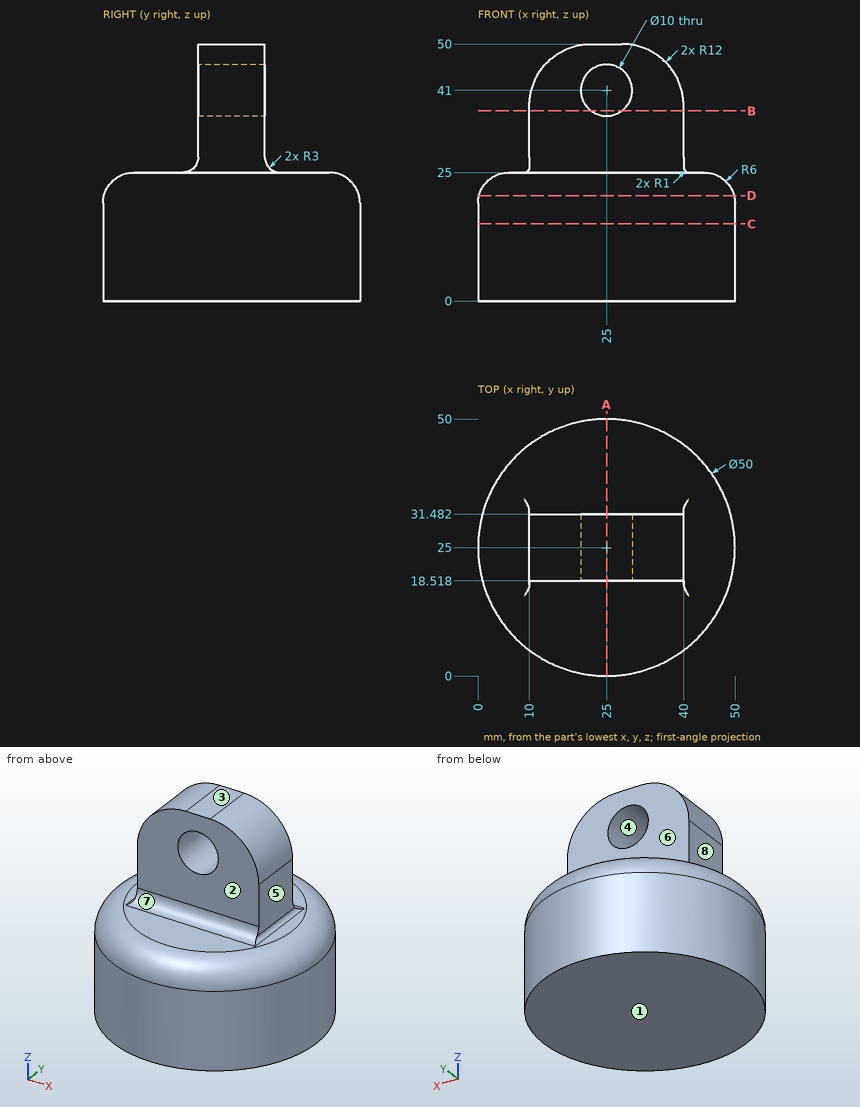
Check sheet for the drawn part. Datum: minimum x, y, z corner. Units: mm. A direction names the side the tool comes from. Give positions to 0.01 mm unless a question says otherwise; leave off trailing zeros. Loops run counter-clockwise (first coordinate to the right, second up) from the corner with the lowest first, then second, coordinate; pieces in that order, holes last. Notation, with made-up numbers: M 39.5,-25 L 52.5,-25 A11 ccw 52.5,-10 Z; hole C 24,-35.5 d10. An arc over 180 degrees is marked long. Return JSON: item names as keys, results as strings.
1) Tool access check on the marked faces 5, 6, 7 and 8. Record the directions out of +Z, -Z, +X, -X, +Y, -Y that give a thin tool (end or side, any length) a straight path to the whole face; none if there is none.
Findings:
{"face 5": "+Z, +X, +Y, -Y", "face 6": "+Z, +X, -X, +Y", "face 7": "+Z, +X, -X, -Y", "face 8": "+Z, -X, +Y, -Y"}
2) Mould release check, pull along Z, two halves, no side actions. Record for the marked faces 1, 2, 3 and 4: released by +Z, released by -Z, zero draft, split by the parting line, or undercut.
Findings:
{"face 1": "released by -Z", "face 2": "zero draft", "face 3": "released by +Z", "face 4": "undercut"}
3) Section check C-C, the plane z = 15. Enter the section's corners in (x, y), and give its area (3 significant figures).
Findings:
{"outline": "C 25,25 d50", "area": "1,960 mm2"}
4) Gauge pin test, flat ends, axial feed: P1, Ø12, axis at y = 15.5, z = 40.5, coming from the +X side; P2, Ø11, axis at x = 31.5, z = 38, coming from the +Y side; P3, Ø10, axis at x = 36, y = 27.5, coming from the -Z side; P4, Ø8, axis at x = 25, z = 41, coming from the -Y side. Record the tip position at first contact, or that the pin passes through.
Findings:
{"P1": "stops at x = 40", "P2": "stops at y = 31.48", "P3": "stops at z = 0", "P4": "passes through"}
5) Section check A-A, the plane x = 25. Enter the section's corners in (y, z).
Findings:
{"outline": "M 0,0 L 50,0 L 50,19 A6 ccw 44,25 L 34.48,25 A3 cw 31.48,28 L 31.48,36 L 18.52,36 L 18.52,28 A3 cw 15.52,25 L 6,25 A6 ccw 0,19 Z; M 18.52,46 L 31.48,46 L 31.48,50 L 18.52,50 Z"}
6) Section check D-D, the plane z = 20.5. Enter the section's corners in (x, y).
Findings:
{"outline": "C 25,25 d49.62"}
7) Material ranges on L1, parallel to X at y = 24.75, z = 41; L2, parallel to Y at x = 25, z = 2.5; L3, parallel to Y at x = 33.5, z = 33, recorded low to high. Write a range as [from, to].
Findings:
{"L1": "x = [10.38, 20], [30, 39.62]", "L2": "y = [0, 50]", "L3": "y = [18.52, 31.48]"}
8) Section check B-B, the plane z = 37. Enter the section's corners in (x, y).
Findings:
{"outline": "M 10,18.52 L 22,18.52 L 22,31.48 L 10,31.48 Z; M 28,18.52 L 40,18.52 L 40,31.48 L 28,31.48 Z"}
